Read the model definition and answer for the solid it produces. Units are mm, in the model's axes. Give positions to 0.01 mm unless a question says otherwise; leave off trailing zeros. Write each loop counter-clockwise with the first axis right and the second up, starting at its lowest first coordinate (ties: lowest second). Pieces come first, ordered by that corner, then holes. Notation, with made-up numbers: (55, 47.25) -> (67, 47.25) arc R10 cw to (67, 63.25) -> close; hole circle Ø9 at (9, 81). An arc over 180 degrees is marked (long way). Put each result on its own line as item: value. Start each with the question number.
from build123d import *

# Parameters (mm, degrees)
SKETCH1_W                      = 69.85
SKETCH1_H                      = 44.45
BOSS_EXTRUDE1_DEPTH            = 3.175
FILLET1_R                      = 6.35
F_6_0_204_DIAMETER_HOLE1_D     = 5.1816
F_6_0_204_DIAMETER_HOLE1_DEPTH = 38.1
F_6_0_204_DIAMETER_HOLE1_TIP   = 1.556709692


with BuildPart() as part:
    # Sketch1 → Boss-Extrude1 (new body)
    with BuildSketch(Plane(origin=(0, 0, 0), x_dir=(1, 0, 0), z_dir=(0, 1, 0))):
        Rectangle(SKETCH1_W, SKETCH1_H)
    extrude(amount=BOSS_EXTRUDE1_DEPTH)

    # Fillet1
    fillet1_edges = [part.edges().sort_by_distance(p)[0] for p in [
        (-34.925, 1.5875, -22.225),
        (34.925, 1.5875, -22.225),
    ]]
    fillet(fillet1_edges, radius=FILLET1_R)

    # #6 (0.204) Diameter Hole1
    with Locations(Plane(origin=(0, 0, 0), x_dir=(-1, 0, 0), z_dir=(0, -1, 0))):
        with Locations((-29.845, 17.78), (29.845, 17.78)):
            Hole(F_6_0_204_DIAMETER_HOLE1_D / 2, depth=F_6_0_204_DIAMETER_HOLE1_DEPTH)
            with Locations((0, 0, -(F_6_0_204_DIAMETER_HOLE1_DEPTH + F_6_0_204_DIAMETER_HOLE1_TIP / 2))):  # 118° drill point
                Cone(0, F_6_0_204_DIAMETER_HOLE1_D / 2, F_6_0_204_DIAMETER_HOLE1_TIP, mode=Mode.SUBTRACT)


solid = part.part
1) A cutting plane is placed at A-A on y = 2. Give the vertices of the cut face in (x, z) (3 decimals).
2) Each of these flat-tipped pins is pushed along its axis until it touches: pin 1 Ø3 at (x, z) = (-29.845, -17.78) entering from -Y; pin 2 Ø1 at (x, z) = (-27, 17) entering from -Y. Where does it stop, or does it pass through?
3) A cutting plane is placed at B-B on z = -17.78. Give the vertices of the cut face in (x, y) (3 decimals).
4) Straight lines are drawn through the part: line 1 (Z direction, x = -29, y = 2.65) (3 decimals); line 2 (X direction, y = 2.5, z = -17.78); line 3 (Z direction, x = 32, y = 0.4) (3 decimals). For each, find the intervals that lie inside material, in ascending order. Write a range as [from, to].
5) For a pull along X with two mould halves and no side action, classify faces 1 (the face through (0, 2, 22.225)), 2 (the face through (-30.18, 1.61, -20.35)), 3 (the face through (-33.11, 1.61, -20.32)) as pulls with the +X half, pulls with the -X half, needs draft (parallel to the pull), parting line crosses it, or undercut.
Results found:
1. outline: (-34.925, -15.875) arc R6.35 ccw to (-28.575, -22.225) -> (28.575, -22.225) arc R6.35 ccw to (34.925, -15.875) -> (34.925, 22.225) -> (-34.925, 22.225) -> close; hole circle Ø5.182 at (-29.845, -17.78); hole circle Ø5.182 at (29.845, -17.78)
2. pin 1: passes through
2. pin 2: stops at y = 0
3. outline: (-34.633, 0) -> (-32.436, 0) -> (-32.436, 3.175) -> (-34.633, 3.175) -> close; (-27.254, 0) -> (27.254, 0) -> (27.254, 3.175) -> (-27.254, 3.175) -> close; (32.436, 0) -> (34.633, 0) -> (34.633, 3.175) -> (32.436, 3.175) -> close
4. line 1: z = [-22.211, -20.229], [-15.331, 22.225]
4. line 2: x = [-34.63, -32.44], [-27.25, 27.25], [32.44, 34.63]
4. line 3: z = [-21.222, -19.218], [-16.342, 22.225]
5. face 1: needs draft
5. face 2: undercut
5. face 3: pulls with the -X half
